from build123d import *

# Parameters (mm, degrees)
F0_R     = 11.0236
F1_DEPTH = 6.35


with BuildPart() as f1:
    # F0 (on Front) → F1 (new body)
    with BuildSketch(Plane.XZ):
        with BuildLine():
            ThreePointArc((0.3671004027, -14.2827831162), (10.2317545723, -9.9721539611), (14.2875, 0))
            ThreePointArc((14.2875, 0), (13.8530020446, 3.4967113981), (12.5759352613, 6.7807454275))
            ThreePointArc((12.5759352613, 6.7807454275), (12.3650513112, 7.1389657031), (12.1602654275, 7.5007066989))
            ThreePointArc((12.1602654275, 7.5007066989), (0.0192332981, 14.2874870544), (-12.1400270316, 7.5334188734))
            ThreePointArc((-12.1400270316, 7.5334188734), (-12.3634468836, 7.1380393864), (-12.5941456375, 6.7468623753))
            ThreePointArc((-12.5941456375, 6.7468623753), (-12.351516996, -7.1814124061), (-0.3671004027, -14.2827831162))
            ThreePointArc((-0.3671004027, -14.2827831162), (0, -14.2800373238), (0.3671004027, -14.2827831162))
        make_face()
        Circle(F0_R, mode=Mode.SUBTRACT)
        with BuildLine():
            ThreePointArc((12.5759352613, 6.7807454275), (13.8530020446, 3.4967113981), (14.2875, 0))
            ThreePointArc((14.2875, 0), (10.2317545723, -9.9721539611), (0.3671004027, -14.2827831162))
            ThreePointArc((0.3671004027, -14.2827831162), (11.7434168793, -17.2721575555), (20.4219768304, -25.2119014612))
            Line((20.4219768304, -25.2119014612), (15.3979316793, -16.51))
            Line((15.3979316793, -16.51), (21.9970452561, -5.08))
            Line((21.9970452561, -5.08), (32.0385831564, -5.08))
            ThreePointArc((32.0385831564, -5.08), (20.8467310821, -1.5462510774), (12.5759352613, 6.7807454275))
        make_face()
        with BuildLine():
            ThreePointArc((12.1602654275, 7.5007066989), (12.3650513112, 7.1389657031), (12.5759352613, 6.7807454275))
            ThreePointArc((12.5759352613, 6.7807454275), (12.3733379566, 7.14375), (12.1602654275, 7.5007066989))
        make_face()
        with BuildLine():
            ThreePointArc((-0.3671004027, -14.2827831162), (0, -14.2875), (0.3671004027, -14.2827831162))
            ThreePointArc((0.3671004027, -14.2827831162), (0, -14.2800373238), (-0.3671004027, -14.2827831162))
        make_face()
        with BuildLine():
            ThreePointArc((-12.1400270316, 7.5334188734), (0.0192332981, 14.2874870544), (12.1602654275, 7.5007066989))
            ThreePointArc((12.1602654275, 7.5007066989), (9.0842728274, 18.8269242417), (11.619882527, 30.2862269147))
            Line((11.619882527, 30.2862269147), (6.5991135768, 21.59))
            Line((6.5991135768, 21.59), (-6.5991135768, 21.59))
            Line((-6.5991135768, 21.59), (-11.617000966, 30.2812359048))
            ThreePointArc((-11.617000966, 30.2812359048), (-9.0824511669, 18.8430392976), (-12.1400270316, 7.5334188734))
        make_face()
        with BuildLine():
            ThreePointArc((35.1952724098, -5.08), (33.6169277831, -5.1308108988), (32.0385831564, -5.08))
            Line((32.0385831564, -5.08), (21.9970452561, -5.08))
            Line((21.9970452561, -5.08), (15.3979316793, -16.51))
            Line((15.3979316793, -16.51), (20.4219768304, -25.2119014612))
            ThreePointArc((20.4219768304, -25.2119014612), (21.2533288946, -26.5506524823), (21.9970452561, -27.94))
            Line((21.9970452561, -27.94), (35.1952724098, -27.94))
            Line((35.1952724098, -27.94), (41.7943859866, -16.51))
            Line((41.7943859866, -16.51), (35.1952724098, -5.08))
        make_face()
        Polygon((33.640814545, -7.7724), (38.6854702571, -16.51), (33.640814545, -25.2476), (23.5515031209, -25.2476), (18.5068474088, -16.51), (23.5515031209, -7.7724), align=None, mode=Mode.SUBTRACT)
        with BuildLine():
            Line((35.1952724098, -5.08), (32.0385831564, -5.08))
            ThreePointArc((32.0385831564, -5.08), (33.6169277831, -5.1308108988), (35.1952724098, -5.08))
        make_face()
        with BuildLine():
            ThreePointArc((-20.4219768304, -25.2119014612), (-11.7434168793, -17.2721575555), (-0.3671004027, -14.2827831162))
            ThreePointArc((-0.3671004027, -14.2827831162), (-12.351516996, -7.1814124061), (-12.5941456375, 6.7468623753))
            ThreePointArc((-12.5941456375, 6.7468623753), (-20.8597762997, -1.5558862096), (-32.0328200345, -5.08))
            Line((-32.0328200345, -5.08), (-21.9970452561, -5.08))
            Line((-21.9970452561, -5.08), (-15.3979316793, -16.51))
            Line((-15.3979316793, -16.51), (-20.4219768304, -25.2119014612))
        make_face()
        with BuildLine():
            ThreePointArc((21.9970452561, -27.94), (21.2533288946, -26.5506524823), (20.4219768304, -25.2119014612))
            Line((20.4219768304, -25.2119014612), (21.9970452561, -27.94))
        make_face()
        with BuildLine():
            ThreePointArc((-12.5941456375, 6.7468623753), (-12.3634468836, 7.1380393864), (-12.1400270316, 7.5334188734))
            ThreePointArc((-12.1400270316, 7.5334188734), (-12.3733379566, 7.14375), (-12.5941456375, 6.7468623753))
        make_face()
        with BuildLine():
            ThreePointArc((13.1982271537, 33.02), (12.3650513112, 31.6785189067), (11.619882527, 30.2862269147))
            Line((11.619882527, 30.2862269147), (13.1982271537, 33.02))
        make_face()
        with BuildLine():
            Line((6.5991135768, 21.59), (11.619882527, 30.2862269147))
            ThreePointArc((11.619882527, 30.2862269147), (12.3650513112, 31.6785189067), (13.1982271537, 33.02))
            Line((13.1982271537, 33.02), (6.5991135768, 44.45))
            Line((6.5991135768, 44.45), (-6.5991135768, 44.45))
            Line((-6.5991135768, 44.45), (-13.1982271537, 33.02))
            ThreePointArc((-13.1982271537, 33.02), (-12.3634468836, 31.6761178835), (-11.617000966, 30.2812359048))
            Line((-11.617000966, 30.2812359048), (-6.5991135768, 21.59))
            Line((-6.5991135768, 21.59), (6.5991135768, 21.59))
        make_face()
        Polygon((10.0893114241, 33.02), (5.0446557121, 24.2824), (-5.0446557121, 24.2824), (-10.0893114241, 33.02), (-5.0446557121, 41.7576), (5.0446557121, 41.7576), align=None, mode=Mode.SUBTRACT)
        with BuildLine():
            ThreePointArc((-21.9970452561, -27.94), (-21.2533288946, -26.5506524823), (-20.4219768304, -25.2119014612))
            Line((-20.4219768304, -25.2119014612), (-15.3979316793, -16.51))
            Line((-15.3979316793, -16.51), (-21.9970452561, -5.08))
            Line((-21.9970452561, -5.08), (-32.0328200345, -5.08))
            ThreePointArc((-32.0328200345, -5.08), (-33.6140462222, -5.1309998622), (-35.1952724098, -5.08))
            Line((-35.1952724098, -5.08), (-41.7943859866, -16.51))
            Line((-41.7943859866, -16.51), (-35.1952724098, -27.94))
            Line((-35.1952724098, -27.94), (-21.9970452561, -27.94))
        make_face()
        Polygon((-23.5515031209, -25.2476), (-33.640814545, -25.2476), (-38.6854702571, -16.51), (-33.640814545, -7.7724), (-23.5515031209, -7.7724), (-18.5068474088, -16.51), align=None, mode=Mode.SUBTRACT)
        with BuildLine():
            Line((-21.9970452561, -27.94), (-20.4219768304, -25.2119014612))
            ThreePointArc((-20.4219768304, -25.2119014612), (-21.2533288946, -26.5506524823), (-21.9970452561, -27.94))
        make_face()
        with BuildLine():
            Line((-13.1982271537, 33.02), (-11.617000966, 30.2812359048))
            ThreePointArc((-11.617000966, 30.2812359048), (-12.3634468836, 31.6761178835), (-13.1982271537, 33.02))
        make_face()
        with BuildLine():
            ThreePointArc((-35.1952724098, -5.08), (-33.6140462222, -5.1309998622), (-32.0328200345, -5.08))
            Line((-32.0328200345, -5.08), (-35.1952724098, -5.08))
        make_face()
    extrude(amount=F1_DEPTH)


solid = f1.part
Input: part model. Units: mm. Frame: model coordinates. A direction names the side the tool comes from. Give positions to 0.01 mm unless a question says otherwise; leave off trailing zeros. Write each loop counter-clockwise with the first axis right and the second up, starting at its lowest first coordinate (ties: lowest second). Pieces come first, ordered by that corner, then holes.
Q1. Pull-direction query (Z, two-part tool) for faces 1 (the face through (29, -3, -27.94)), 2 (the face through (-34, -3, -5.08)), 3 (the face through (20.994, -3.131, -12.202)); classes: pulls with the +Z half, pulls with the -Z half, needs draft (parallel to the pull), parting line crosses it, or undercut.
Q2. Section A-A, the plane x = -8. Output: boundary loops of the cut face in (y, z), plus the area to 3 significant figures.
Q3. Section B-B, the plane z = 0. Output: boundary loops of the cut face in (x, y).
Q4. Section D-D, the plane z = 17.5. Output: boundary loops of the cut face in (x, y), plus the area to 3 significant figures.
Q5. Material intervals for probe 1 along Z at (x, y) = (0, -3.5); probe 2 along X at (y, z) = (-2.5, -9.5); probe 3 along X at (y, z) = (-5.5, -19.5), sorted ascending.
Q6. First-contact query: P1, Ø1.9, axis at x = 31, y = -3.5, coming from the +Z side; P2, Ø0.9, axis at x = -34.5, y = -3.5, coming from the +Z side; P3, Ø3, axis at x = -29, y = -3, coming from the +Z side; P4, Ø13, axis at x = 0, z = 0, coming from the -Y side. Flat tips, straight axial feed; report the tip coordinate or a pass-through.
Q7. Set-up query: faces 4 (the face through (36.13, -3.13, -12.08)), 5 (the face through (-11.889, -3.131, -17.352)), 6 (the face through (12.398, -3.131, 31.634)). Return all of +Z, -Z, +X, -X, +Y, -Y with unobstructed straight access to the full face (end or side cutting, diameter ignored); none if empty.
Q8. Section C-C, the plane y = -2.5. State how many separate pieces and enclosed holes the cut face has, plus the area to 3 significant figures.
Filled in:
1. face 1: pulls with the -Z half
1. face 2: pulls with the +Z half
1. face 3: undercut
2. outline: (-6.35, -15.62) - (0, -15.62) - (0, -7.58) - (-6.35, -7.58) - close; (-6.35, 7.58) - (0, 7.58) - (0, 29.4) - (-6.35, 29.4) - close; (-6.35, 36.64) - (0, 36.64) - (0, 42.02) - (-6.35, 42.02) - close
2. area: 224 mm2
3. outline: (-18.6, -6.35) - (-11.02, -6.35) - (-11.02, 0) - (-18.6, 0) - close; (11.02, -6.35) - (18.6, -6.35) - (18.6, 0) - (11.02, 0) - close
4. outline: (-9.15, -6.35) - (9.15, -6.35) - (9.15, 0) - (-9.15, 0) - close
4. area: 116 mm2
5. probe 1: z = -14.29 to -11.02, 11.02 to 24.28, 41.76 to 44.45
5. probe 2: x = -37.75 to -34.64, -22.55 to -5.59, 5.59 to 22.55, 34.64 to 37.75
5. probe 3: x = -40.07 to -36.96, -20.23 to -15.13, 15.13 to 20.23, 36.96 to 40.07
6. P1: stops at z = -4.87
6. P2: stops at z = -5.08
6. P3: stops at z = -4.36
6. P4: passes through
7. face 4: +Y, -Y
7. face 5: -Z, +Y, -Y
7. face 6: +X, +Y, -Y
8. separate pieces: 1
8. enclosed holes: 4
8. area: 1,370 mm2
